```python
from build123d import *

# Parameters (mm, degrees)
SKETCH1_R           = 9
SKETCH1_R_2         = 2.2
BOSS_EXTRUDE1_DEPTH = 7
SKETCH2_R           = 9
SKETCH2_R_2         = 5.5
CUT_EXTRUDE1_DEPTH  = 3.8
SKETCH3_R           = 5.5
SKETCH3_R_2         = 3.875
CUT_EXTRUDE2_DEPTH  = 3


with BuildPart() as part:
    # Sketch1 → Boss-Extrude1 (new body)
    with BuildSketch(Plane.XY):
        Circle(SKETCH1_R)
        Circle(SKETCH1_R_2, mode=Mode.SUBTRACT)
    extrude(amount=BOSS_EXTRUDE1_DEPTH)

    # Sketch2 → Cut-Extrude1 (cut)
    with BuildSketch(Plane.XY.offset(7)):
        Circle(SKETCH2_R)
        Circle(SKETCH2_R_2, mode=Mode.SUBTRACT)
    extrude(amount=-CUT_EXTRUDE1_DEPTH, mode=Mode.SUBTRACT)

    # Sketch3 → Cut-Extrude2 (cut)
    with BuildSketch(Plane.XY.offset(7)):
        Circle(SKETCH3_R)
        Circle(SKETCH3_R_2, mode=Mode.SUBTRACT)
    extrude(amount=-CUT_EXTRUDE2_DEPTH, mode=Mode.SUBTRACT)


solid = part.part
```
The model under review builds one solid part; all positions refer to its coordinate system, in mm. A direction names the side the tool comes from. Coordinates: 2 decimals unless noted, no trailing zeros. Order: outer loops, then holes, each group sorted by start corner. A loop starts at its lowest first (then second) coordinate and runs counter-clockwise, first axis right, second up. Notation, with made-up numbers: M -26,23.5 L -16,23.5 A30 ccw -16,55.5 Z; hole C 13,-20.5 d10. An arc over 180 degrees is marked long. One line per question, with ' | ' between items.
(1) Add section A-A, the plane x = 0. Write out the cut boundary in (y, z) (3 decimals).
Geometry results:
outline: M -9,0 L -2.2,0 L -2.2,7 L -3.875,7 L -3.875,4 L -5.5,4 L -5.5,3.2 L -9,3.2 Z; M 2.2,0 L 9,0 L 9,3.2 L 5.5,3.2 L 5.5,4 L 3.875,4 L 3.875,7 L 2.2,7 Z
(2) Insertion check: pin 1 (2.5 mm diameter, centred on x = 0, y = 0, fed in from +Z); pin 2 (3 mm diameter, centred on y = -6.5, z = 1, fed in from -X). Each pin has a flat end and moves straight along its axis. Give the tip position at first contact, or say it passes through.
Geometry results:
pin 1: passes through | pin 2: stops at x = -7.48
(3) For probe 1 along Y at (x, z) = (0, 2.25); probe 2 along Y at (x, z) = (0, 3.25); probe 3 along Z at (x, y) = (2, -7.5), list the stretches that pass through material, from the lowest coordinate up. Write a range as from..to.
Geometry results:
probe 1: y = -9..-2.2, 2.2..9 | probe 2: y = -5.5..-2.2, 2.2..5.5 | probe 3: z = 0..3.2
(4) Machinability: for faces 4 (the face through (-1.19, -5.37, 3.61)), 5 (the face through (2, -2, 7)), which of the approach directions +Z, -Z, +X, -X, +Y, -Y give a long, thin tool a straight path to every point of the face, cutting with its end or side? Answer none if there is none.
Geometry results:
face 4: +Z | face 5: +Z, +X, -X, +Y, -Y
(5) The part is to be moulded in two halves that separate along X. For faces 1 (the face through (2, -2, 0)), 2 (the face through (-0.504, 3.842, 5.521)), 3 (the face through (2.1, 0.66, 3.45)), say which applies: +X half, -X half, draft (parallel to the pull), parting line (faces both ways), or undercut.
Geometry results:
face 1: draft | face 2: parting line | face 3: undercut
(6) Add section D-D, the plane x = 3.5. Write out the cut boundary in (y, z), then the cut area to 3 significant figures.
Geometry results:
outline: M -8.29,0 L 8.29,0 L 8.29,3.2 L 4.24,3.2 L 4.24,4 L 1.66,4 L 1.66,7 L -1.66,7 L -1.66,4 L -4.24,4 L -4.24,3.2 L -8.29,3.2 Z | area: 69.8 mm²
(7) Add section C-C, the plane z = 2. Write out the cut boundary in (x, y).
Geometry results:
outline: C 0,0 d18; hole C 0,0 d4.4
